Could you check a few things on this model? Use its own coordinates, in mm. Face numbers are marked on the shaded views. A direction names the side the tool comes from. Coordinates: 2 decimals unless noted, no trailing zeros. Write each loop counter-clockwise with the first axis right and the second up, starting at its lowest first coordinate (ties: lowest second). Pieces come first, ordered by that corner, then holes.
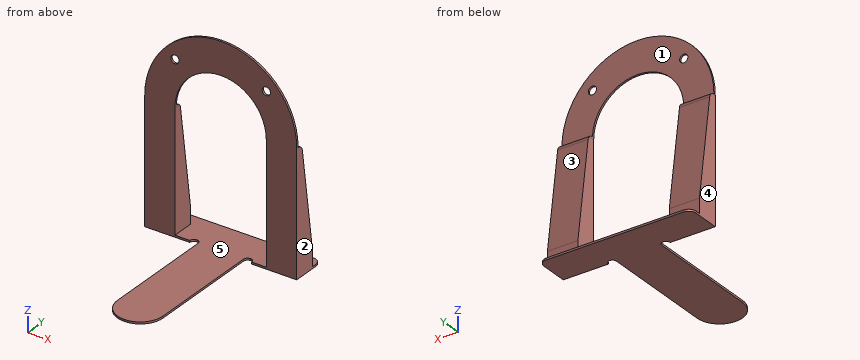
```python
from build123d import *

# Parameters (mm, degrees)
F1_DEPTH = 126.746
F3_DEPTH = 1.6012
F4_R     = 3.429
F5_DEPTH = 28.9316
F7_DEPTH = 25.4


with BuildPart() as f1:
    # F0 (on Right) → F1 (new body)
    with BuildSketch(Plane.YZ):
        with BuildLine():
            Line((16.653205, 65.313007), (15.053005, 65.313007))
            Line((15.053005, 65.313007), (15.053005, -19.597488))
            Line((15.053005, -19.597488), (15.053005, -99.786993))
            Line((15.053005, -99.786993), (-99.246995, -99.786993))
            Line((-99.246995, -99.786993), (-99.246995, -101.387193))
            Line((-99.246995, -101.387193), (43.983605, -101.387193))
            Line((43.983605, -101.387193), (43.983605, -99.786993))
            Line((43.983605, -99.786993), (33.849005, -99.786993))
            Line((33.849005, -99.786993), (33.849005, -87.752856))
            Line((33.849005, -87.752856), (21.68237, -2.397729))
            ThreePointArc((21.68237, -2.397729), (19.982223, 0.722598), (16.653205, 1.965407))
            Line((16.653205, 1.965407), (16.653205, 65.313007))
        make_face()
    extrude(amount=F1_DEPTH)

    # F2 (on face) → F3 (cut, through all)
    with BuildSketch(Plane.XY.offset(-99.786993)):
        with BuildLine():
            Line((0, -99.246995), (63.246, -99.246995))
            ThreePointArc((63.246, -99.246995), (49.955221, -93.741774), (44.45, -80.450995))
            Line((44.45, -80.450995), (44.45, 15.053005))
            Line((44.45, 15.053005), (0, 15.053005))
            Line((0, 15.053005), (0, -99.246995))
        make_face()
        with BuildLine():
            ThreePointArc((82.296, -80.450995), (76.790779, -93.741774), (63.5, -99.246995))
            Line((63.5, -99.246995), (126.746, -99.246995))
            Line((126.746, -99.246995), (126.746, 15.053005))
            Line((126.746, 15.053005), (82.296, 15.053005))
            Line((82.296, 15.053005), (82.296, -80.450995))
        make_face()
    extrude(amount=-F3_DEPTH, mode=Mode.SUBTRACT)

    # F4 (on face) → F5 (cut, through all)
    with BuildSketch(Plane.XZ.offset(-15.053005)):
        with BuildLine():
            Line((0, 65.313007), (0, 2.067007))
            ThreePointArc((0, 2.067007), (18.524325, 46.788682), (63.246, 65.313007))
            Line((63.246, 65.313007), (0, 65.313007))
        make_face()
        with BuildLine():
            Line((126.746, 65.313007), (63.5, 65.313007))
            ThreePointArc((63.5, 65.313007), (108.221675, 46.788682), (126.746, 2.067007))
            Line((126.746, 2.067007), (126.746, 65.313007))
        make_face()
        with BuildLine():
            Line((25.146, 0.365207), (25.146, -99.786993))
            Line((25.146, -99.786993), (44.45, -99.786993))
            Line((44.45, -99.786993), (82.296, -99.786993))
            Line((82.296, -99.786993), (101.346, -99.786993))
            Line((101.346, -99.786993), (101.346, 0.365207))
            ThreePointArc((101.346, 0.365207), (90.186768, 27.305975), (63.246, 38.465207))
            ThreePointArc((63.246, 38.465207), (36.305232, 27.305975), (25.146, 0.365207))
        make_face()
        with Locations((25.146, 38.465207)):
            Circle(F4_R)
        with Locations((101.346, 38.465207)):
            Circle(F4_R)
    extrude(amount=-F5_DEPTH, mode=Mode.SUBTRACT)

    # F6 (on face) → F7 (cut)
    with BuildSketch(Plane(origin=(0, 0, -101.387193), x_dir=(1, 0, 0), z_dir=(0, 0, -1))):
        with BuildLine():
            ThreePointArc((6.35, -43.983605), (1.859872, -42.123733), (0, -37.633605))
            Line((0, -37.633605), (0, -43.983605))
            Line((0, -43.983605), (6.35, -43.983605))
        make_face()
        with BuildLine():
            ThreePointArc((37.592, -15.053005), (38.596331, -17.477674), (41.021, -18.482005))
            ThreePointArc((41.021, -18.482005), (43.445669, -17.477674), (44.45, -15.053005))
            Line((44.45, -15.053005), (37.592, -15.053005))
        make_face()
        with BuildLine():
            Line((89.154, -15.053005), (82.296, -15.053005))
            ThreePointArc((82.296, -15.053005), (83.300331, -17.477674), (85.725, -18.482005))
            ThreePointArc((85.725, -18.482005), (88.149669, -17.477674), (89.154, -15.053005))
        make_face()
        with BuildLine():
            ThreePointArc((126.746, -37.633605), (124.886128, -42.123733), (120.396, -43.983605))
            Line((120.396, -43.983605), (126.746, -43.983605))
            Line((126.746, -43.983605), (126.746, -37.633605))
        make_face()
    extrude(amount=-F7_DEPTH, mode=Mode.SUBTRACT)


solid = f1.part
```
1. I want a section at D-D on x = 8.5. Please give me the cut outline in (y, z).
Verdict:
outline: (15.05, -101.39) - (43.98, -101.39) - (43.98, -99.79) - (33.85, -99.79) - (33.85, -87.75) - (21.68, -2.4) arc R5.08 ccw to (16.65, 1.97) - (16.65, 33.74) - (15.05, 33.74) - close
2. I want a section at C-C on y = 26.5. Please give me the cut outline in (x, z), plus the area to 3 significant figures.
Verdict:
outline: (0, -101.39) - (126.75, -101.39) - (126.75, -36.2) - (101.35, -36.2) - (101.35, -99.79) - (25.15, -99.79) - (25.15, -36.2) - (0, -36.2) - close
area: 3,420 mm2
3. Please list where these lines run through material, in increasing order: line 1 along X through (y, z) = (16.5, -9); line 2 along Z through (x, y) = (81.5, -76.5); line 3 along Y through (x, z) = (72.5, 57).
Verdict:
line 1: x = 0 to 25.15, 101.35 to 126.75
line 2: z = -101.39 to -99.79
line 3: y = 15.05 to 16.65
4. For pin 1 (1 mm diameter, centred on x = 105.5, z = 35.5, fed in from -Y); pin 2 (6 mm diameter, centred on x = 16.5, z = 13, fed in from +Y); pin 3 (1.3 mm diameter, centred on y = -17.5, z = -100, fed in from +X); pin 4 (5.5 mm diameter, centred on x = 101.35, z = 38.47, fed in from +Y), each with a flat end and sliding along its axis, tell me the tip position at first contact or that it passes through.
Verdict:
pin 1: stops at y = 15.05
pin 2: stops at y = 16.65
pin 3: stops at x = 82.3
pin 4: passes through
5. I want a section at B-B on z = 10.5. Please give me the cut outline in (x, y).
Verdict:
outline: (0.56, 15.05) - (26.52, 15.05) - (26.52, 16.65) - (0.56, 16.65) - close; (99.97, 15.05) - (126.18, 15.05) - (126.18, 16.65) - (99.97, 16.65) - close
6. I want a section at A-A on x = 59.5. Please give me the cut outline in (y, z).
Verdict:
outline: (-98.87, -101.39) - (43.98, -101.39) - (43.98, -99.79) - (-98.87, -99.79) - close; (15.05, 38.28) - (16.65, 38.28) - (16.65, 65.2) - (15.05, 65.2) - close
7. If we mould it in two halves opening along X, with no side actions, what happens to the marked faces 3, 4 and 5? For each: pulls with the +X half, pulls with the -X half, needs draft (parallel to the pull), parting line crosses it, or undercut.
Verdict:
face 3: needs draft
face 4: pulls with the -X half
face 5: undercut
8. On a 3-axis mill with a long thin cutter (end or side, diameter ignored), from which of +Z, -Z, +X, -X, +Y, -Y can I reach the whole of each face in a straight line? I mean the marked faces 1 and 2. Say none if no direction works.
Verdict:
face 1: +Z, +X, -X, +Y
face 2: +Z, -Z, +X, +Y, -Y
